Here's how the part is built. I have some questions about the finished solid (model axes, mm). Face numbers are marked on the shaded views. A direction names the side the tool comes from. Round coordinates to 2 decimals unless told otherwise and drop trailing zeros. Order: outer loops, then holes, each group sorted by start corner. A loop starts at its lowest first (then second) coordinate and runs counter-clockwise, first axis right, second up. Notation, with made-up numbers: (-37, 32.25) - (16, 32.25) arc R13 cw to (16, 54.25) - close; hole circle Ø6 at (30.5, 67). An arc over 180 degrees is marked (long way). One line per item, written item: value.
from build123d import *

# Parameters (mm, degrees)
SKETCH1_W           = 7
SKETCH1_H           = 13.6
BOSS_EXTRUDE1_DEPTH = 7.95
SKETCH2_W           = 8.89
SKETCH2_H           = 21.59
SKETCH2_R           = 1.5
SKETCH2_R_2         = 0.325
BOSS_EXTRUDE2_DEPTH = 0.6


with BuildPart() as part:
    # Sketch1 → Boss-Extrude1 (new body)
    with BuildSketch(Plane(origin=(0, 0, 0), x_dir=(1, 0, 0), z_dir=(0, 1, 0))):
        Rectangle(SKETCH1_W, SKETCH1_H)
    extrude(amount=BOSS_EXTRUDE1_DEPTH)

    # Sketch2 → Boss-Extrude2 (add)
    with BuildSketch(Plane.XZ):
        with Locations((0.029445322, -0.999566393)):
            Rectangle(SKETCH2_W, SKETCH2_H)
        with Locations(Location((0.01501125, -9.254566393, 0), (0, 0, 270))):
            Circle(SKETCH2_R, mode=Mode.SUBTRACT)
        with Locations(Location((0.029445322, 8.376560571, 0), (0, 0, 270))):
            Circle(SKETCH2_R_2, mode=Mode.SUBTRACT)
        with Locations(Location((2.569445322, 8.376560571, 0), (0, 0, 270))):
            Circle(SKETCH2_R_2, mode=Mode.SUBTRACT)
        with Locations(Location((-2.510554678, 8.376560571, 0), (0, 0, 270))):
            Circle(SKETCH2_R_2, mode=Mode.SUBTRACT)
    extrude(amount=BOSS_EXTRUDE2_DEPTH)


solid = part.part
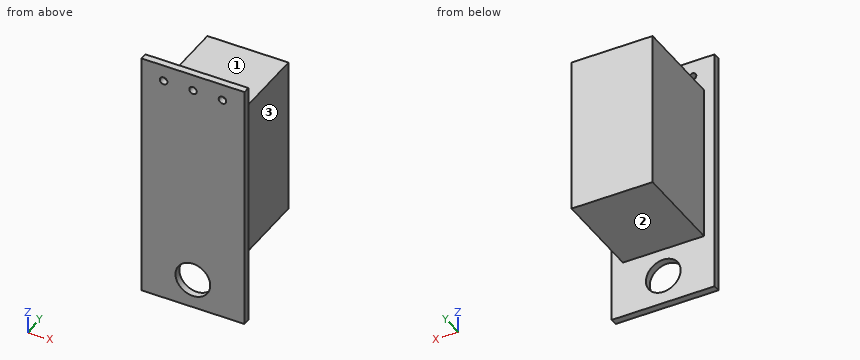
Q1. If we section it at D-D, the plane y = 7.5: Please give me the cut outline in (x, z), then the cut area to 3 significant figures.
Results list:
outline: (-3.5, -6.8) - (3.5, -6.8) - (3.5, 6.8) - (-3.5, 6.8) - close
area: 95.2 mm²
Q2. If we section it at C-C, the plane z = 5.25: Please give me the cut outline in (x, y).
Results list:
outline: (-4.42, -0.6) - (4.47, -0.6) - (4.47, 0) - (3.5, 0) - (3.5, 7.95) - (-3.5, 7.95) - (-3.5, 0) - (-4.42, 0) - close
Q3. If I drill on line 1 along Z through (x, y) = (3.25, 1.5); line 2 along X through (y, z) = (3.25, 5.5); line 3 along Y through (x, z) = (4, 5.25), over which ranges is the centre line in solid material (lowest first)?
Results list:
line 1: -6.8 to 6.8
line 2: -3.5 to 3.5
line 3: -0.6 to 0
Q4. Which directions (+Z, -Z, +X, -X, +Y, -Y) give clear straight access to the entire face, cutting with the end or side of a thin tool? Please do the marked faces 1, 2 and 3.
Results list:
face 1: +Z, +X, -X, +Y
face 2: -Z, +X, -X, +Y
face 3: +Z, -Z, +X, +Y
Q5. Will these pins go through, and if not, where does the flat tip stop? pin 1 (3 mm diameter, centred on y = 2.5, z = -5, fed in from +X); pin 2 (1 mm diameter, centred on x = -1, y = 2, fed in from -Z); pin 3 (4 mm diameter, centred on y = 5, z = 1, fed in from -X).
Results list:
pin 1: x = 3.5
pin 2: z = -6.8
pin 3: x = -3.5
Q6. If we section it at B-B, the plane z = 8.5: Please give me the cut outline in (x, y), then the cut area to 3 significant figures.
Results list:
outline: (-4.42, -0.6) - (-2.81, -0.6) - (-2.81, 0) - (-4.42, 0) - close; (-2.21, -0.6) - (-0.27, -0.6) - (-0.27, 0) - (-2.21, 0) - close; (0.33, -0.6) - (2.27, -0.6) - (2.27, 0) - (0.33, 0) - close; (2.87, -0.6) - (4.47, -0.6) - (4.47, 0) - (2.87, 0) - close
area: 4.25 mm²
Q7. If we section it at A-A, the plane x = -1: Please give me the cut outline in (y, z).
Results list:
outline: (-0.6, -11.79) - (0, -11.79) - (0, -10.36) - (-0.6, -10.36) - close; (-0.6, -8.15) - (0, -8.15) - (0, -6.8) - (7.95, -6.8) - (7.95, 6.8) - (0, 6.8) - (0, 9.8) - (-0.6, 9.8) - close
